Read the model definition and answer for the solid it produces. Units are mm, in the model's axes. A direction names the side the tool comes from. Coordinates: 2 decimals unless noted, no trailing zeros. Order: outer loops, then holes, each group sorted by start corner. A loop starts at its lowest first (then second) coordinate and runs counter-clockwise, first axis right, second up. Notation, with made-up numbers: M 84.5,75 L 115.5,75 A32 cw 115.5,112 Z; hole C 29,46 d6. An arc over 180 degrees is marked long. Use a Markdown table: item, result. Add a question column.
1) Find section A-A on y = 20.5. Write down the section's boundary in (x, z).
2) The mould has two halves that part along X. Classify faces 3 (the face through (99, 25, -3)), 4 (the face through (0, 23, -36)), 5 (the face through (97, 0, -37)): released by +X, released by -X, zero draft, split by the parting line, or undercut.
3) Find section B-B on z = -6.5. Write down the section's boundary in (x, y), plus the area to 3 significant figures.
4) Each of these flat-tipped pins is pushed along its axis until it touches: pin 1 Ø0.9 at (x, z) = (194, -64) entering from -Y; pin 2 Ø2 at (x, z) = (152, -46) entering from +Y. Where does it stop, or does it pass through?
5) Find the intervals of material crossed by probe 1 along Z at (x, y) = (160.5, 29.5); probe 2 along X at (y, z) = (37, -41.5); probe 3 along Y at (x, z) = (77.5, -44), in increasing order. Write a range as [from, to].
6) For faces 1 (the face through (97, 23, 0)), 2 (the face through (193, 30, -36)), determine the directions among +Z, -Z, +X, -X, +Y, -Y from which every point of the face is accessible in a straight line to the end or side of a thin tool.
7) Find section C-C on y = 43. Write down the section's boundary in (x, z).
8) Find section D-D on x = 29. Write down the section's boundary in (y, z).
from build123d import *

# Parameters (mm, degrees)
SKETCH1_W           = 196
SKETCH1_H           = 73
BOSS_EXTRUDE1_DEPTH = 3
SKETCH3_W           = 196
SKETCH3_H           = 73
SKETCH3_W_2         = 190
SKETCH3_H_2         = 67
BOSS_EXTRUDE2_DEPTH = 44
FILLET1_R           = 1
SKETCH4_W           = 12
SKETCH4_H           = 23
CUT_EXTRUDE1_DEPTH  = 197


with BuildPart() as part:
    # Sketch1 → Boss-Extrude1 (new body)
    with BuildSketch(Plane(origin=(0, 0, 0), x_dir=(1, 0, 0), z_dir=(0, 1, 0))):
        with Locations((98, 36.5)):
            Rectangle(SKETCH1_W, SKETCH1_H)
    extrude(amount=BOSS_EXTRUDE1_DEPTH)

    # Sketch3 → Boss-Extrude2 (add)
    with BuildSketch(Plane(origin=(0, 3, 0), x_dir=(1, 0, 0), z_dir=(0, 1, 0))):
        with Locations((98, 36.5)):
            Rectangle(SKETCH3_W, SKETCH3_H)
        with Locations((98, 36.5)):
            Rectangle(SKETCH3_W_2, SKETCH3_H_2, mode=Mode.SUBTRACT)
    extrude(amount=BOSS_EXTRUDE2_DEPTH)

    # Fillet1
    fillet1_edges = [part.edges().sort_by_distance(p)[0] for p in [
        (0, 23.5, -73),
        (196, 23.5, -73),
        (196, 23.5, 0),
        (0, 23.5, 0),
    ]]
    fillet(fillet1_edges, radius=FILLET1_R)

    # Sketch4 → Cut-Extrude1 (cut, through all)
    with BuildSketch(Plane(origin=(196, 0, 0), x_dir=(0, 0, -1), z_dir=(1, 0, 0))):
        with Locations((9, 14.5)):
            Rectangle(SKETCH4_W, SKETCH4_H)
        with Locations((64, 14.5)):
            Rectangle(SKETCH4_W, SKETCH4_H)
    extrude(amount=-CUT_EXTRUDE1_DEPTH, mode=Mode.SUBTRACT)


solid = part.part
Check result:
| question | item | result |
|---|---|---|
| 1 | outline | M 0,-72 A1 ccw 1,-73 L 195,-73 A1 ccw 196,-72 L 196,-70 L 0,-70 Z; M 0,-58 L 3,-58 L 3,-15 L 0,-15 Z; M 0,-3 L 196,-3 L 196,-1 A1 ccw 195,0 L 1,0 A1 ccw 0,-1 Z; M 193,-58 L 196,-58 L 196,-15 L 193,-15 Z |
| 2 | face 3 | undercut |
| 2 | face 4 | released by -X |
| 2 | face 5 | zero draft |
| 3 | outline | M 0,0 L 196,0 L 196,3 L 0,3 Z; M 0,26 L 3,26 L 3,47 L 0,47 Z; M 193,26 L 196,26 L 196,47 L 193,47 Z |
| 3 | area | 714 mm2 |
| 4 | pin 1 | stops at y = 0 |
| 4 | pin 2 | stops at y = 3 |
| 5 | probe 1 | z = [-73, -70], [-3, 0] |
| 5 | probe 2 | x = [0, 3], [193, 196] |
| 5 | probe 3 | y = [0, 3] |
| 6 | face 1 | +Z, +X, -X, +Y, -Y |
| 6 | face 2 | +Y |
| 7 | outline | M 0,-72 A1 ccw 1,-73 L 195,-73 A1 ccw 196,-72 L 196,-1 A1 ccw 195,0 L 1,0 A1 ccw 0,-1 Z; hole M 3,-70 L 193,-70 L 193,-3 L 3,-3 Z |
| 8 | outline | M 0,-73 L 47,-73 L 47,-70 L 3,-70 L 3,-3 L 47,-3 L 47,0 L 0,0 Z |
